from build123d import *
from build123d.topology import SkipClean

# Parameters (mm, degrees)
SKETCH_1_R               = 12.75
EXTRUDE_1_DEPTH          = 7
EXTRUDE_START            = -2.3
SKETCH_1_3_R             = 12.75
SKETCH_1_3_R_2           = 9.75
EXTRUDE_2_DEPTH          = 2.3
EXTRUDE_3_DEPTH          = 3.3
FILLET_1_R               = 1
EXTRUDE_4_DEPTH          = 3.3
CUT_EXTRUDE_1_REACH      = 22.288
SKETCH_6_R               = 1.3500000000000005
SKETCH_6_R_2             = 1.5499999999999994
CUT_EXTRUDE_START        = -1
CUT_EXTRUDE_2_DEPTH      = 1
EXTRUDE_START_2          = 4.5
EXTRUDE_5_DEPTH          = 4.5
CUT_EXTRUDE_3_DEPTH      = 3
CUT_EXTRUDE_3_DEPTH_BACK = 25
SKETCH_17_R              = 2.5
SKETCH_17_R_2            = 2.5000000000000004
CUT_EXTRUDE_4_DEPTH      = 6.3
SKETCH_18_R              = 2.1
CUT_EXTRUDE_5_DEPTH      = 19.000000000000004


with BuildPart() as part:
    # 草图1 → 凸台-拉伸1 (new body)
    with BuildSketch(Plane(origin=(0, 0, 0), x_dir=(0, 0, -1), z_dir=(1, 0, 0))):
        Circle(SKETCH_1_R)
    extrude(amount=EXTRUDE_1_DEPTH)

    # 草图1<3> → 凸台-拉伸2 (add)
    with BuildSketch(Plane(origin=(0, 0, 0), x_dir=(0, 0, -1), z_dir=(1, 0, 0)).offset(EXTRUDE_START)):
        Circle(SKETCH_1_3_R)
        Circle(SKETCH_1_3_R_2, mode=Mode.SUBTRACT)
    extrude(amount=EXTRUDE_2_DEPTH)

    # 草图4 → 凸台-拉伸3 (add)
    with BuildSketch(Plane(origin=(7, 0, 0), x_dir=(0, 0, -1), z_dir=(1, 0, 0))):
        with BuildLine():
            Line((7.293731545630563, -1.9503794862215074), (5.5903528728314456, -1.4948876985254207))
            ThreePointArc((5.590352872831452, -1.4948876985253963), (4.450095710648993, -0.01722480337626947), (5.557231396787749, 1.4854144081735148))
            ThreePointArc((5.557231396787749, 1.4854144081735148), (5.599745988830406, 1.4974300406171406), (5.642585759719926, 1.508229114174971))
            Line((5.642585759719926, 1.5082291141749726), (7.293933423650666, 1.949624376989515))
            ThreePointArc((7.293933423650662, 1.949624376989514), (4.6e-16, 7.550000000000002), (-7.293933423650662, 1.949624376989515))
            Line((-7.293933423650666, 1.949624376989515), (-5.642585759719924, 1.5082291141749722))
            ThreePointArc((-5.642585759719924, 1.5082291141749706), (-5.599745988830406, 1.4974300406171406), (-5.557231396787749, 1.4854144081735148))
            ThreePointArc((-5.557231396787749, 1.4854144081735148), (-4.757262832498563, 0.9263392102844973), (-4.449999999999999, 0))
            ThreePointArc((-4.449999999999999, -3.8e-16), (-4.767633770522892, -0.9400922701758461), (-5.590352872831452, -1.4948876985253963))
            Line((-5.5903528728314456, -1.4948876985254207), (-7.293731545630563, -1.9503794862215074))
            ThreePointArc((-7.2937315456305605, -1.950379486221506), (-1.39e-15, -7.550000000000002), (7.2937315456305605, -1.9503794862215056))
        make_face()
        with BuildLine():
            ThreePointArc((-0.9205316546017519, -3.4285742624123157), (-1.7750000000000141, -3.074390183434749), (-2.5089665827097076, -2.5114909290789753))
            ThreePointArc((-2.5089665827097076, -2.5114909290789753), (-2.5295691102475106, -2.490738869589025), (-2.55, -2.4698178070456938))
            Line((-2.55, -2.4698178070456938), (-2.55, 0))
            Line((-2.55, 0), (-2.55, 2.4698178070456938))
            ThreePointArc((-2.55, 2.469817807045694), (2.2e-16, 3.5499999999999994), (2.55, 2.4698178070456938))
            Line((2.55, 2.4698178070456938), (2.55, -1.2e-16))
            Line((2.55, -1.2e-16), (2.55, -2.4698178070456938))
            ThreePointArc((2.549999999999999, -2.4698178070456946), (0.9453016753082151, -3.4218276903811913), (-0.9205316546017519, -3.4285742624123157))
        make_face(mode=Mode.SUBTRACT)
    extrude(amount=EXTRUDE_3_DEPTH)

    # 圆角1
    fillet_1_edges = [part.edges().sort_by_distance(p)[0] for p in [
        (7, 1.56e-15, 12.75),
    ]]
    fillet(fillet_1_edges, radius=FILLET_1_R)

    # 草图5 → 凸台-拉伸4 (add)
    with BuildSketch(Plane(origin=(7, 0, 0), x_dir=(0, 0, -1), z_dir=(1, 0, 0))):
        with BuildLine():
            ThreePointArc((5.65345654698472, -1.3047634403110198), (4.6499999999999995, 1.7e-16), (5.65345654698472, 1.3047634403110198))
            Line((5.65345654698472, 1.3047634403110195), (7.3500000000000005, 1.7553631492193538))
            Line((7.3500000000000005, 1.7553631492193538), (7.293933423650666, 1.9496243769895145))
            Line((7.293933423650666, 1.9496243769895145), (5.642585759719882, 1.5082291141749606))
            ThreePointArc((5.642585759719882, 1.5082291141749606), (4.4500975021885605, 0.01738526036219645), (5.60884432582712, -1.499832403491257))
            Line((5.60884432582712, -1.499832403491257), (7.293731545630563, -1.950379486221502))
            Line((7.293731545630563, -1.950379486221502), (7.3500000000000005, -1.7595376594411802))
            Line((7.3500000000000005, -1.7595376594411802), (5.65345654698472, -1.3047634403110195))
        make_face()
    extrude(amount=EXTRUDE_4_DEPTH)

    # 草图6 → 切除-拉伸1 (cut, up to next)
    with BuildSketch(Plane(origin=(7, 0, 0), x_dir=(0, 0, -1), z_dir=(1, 0, 0)), mode=Mode.PRIVATE) as cut_extrude_1_sk1:
        with Locations(Location((6, 0, 0), (0, 0, 255.125726416))):
            Circle(SKETCH_6_R)
    cut_extrude_1_tool1 = extrude(cut_extrude_1_sk1.sketch, amount=-CUT_EXTRUDE_1_REACH, mode=Mode.PRIVATE) & part.part
    # 草图6 → 切除-拉伸1 (cut, up to next)
    with BuildSketch(Plane(origin=(7, 0, 0), x_dir=(0, 0, -1), z_dir=(1, 0, 0)), mode=Mode.PRIVATE) as cut_extrude_1_sk2:
        with Locations(Location((-6, -7.3e-16, 0), (0, 0, 76.668199875))):
            Circle(SKETCH_6_R_2)
    cut_extrude_1_tool2 = extrude(cut_extrude_1_sk2.sketch, amount=-CUT_EXTRUDE_1_REACH, mode=Mode.PRIVATE) & part.part
    add(cut_extrude_1_tool1.solids().sort_by_distance((7, 0, -6))[0], mode=Mode.SUBTRACT)
    add(cut_extrude_1_tool2.solids().sort_by_distance((7, 0, 6))[0], mode=Mode.SUBTRACT)

    # 草图7 → 切除-拉伸2 (cut)
    with BuildSketch(Plane(origin=(7, 0, 0), x_dir=(0, 0, -1), z_dir=(1, 0, 0)).offset(CUT_EXTRUDE_START)):
        with BuildLine():
            Line((2.55, -2.4698178070456938), (2.55, 2.4698178070456938))
            ThreePointArc((2.55, 2.4698178070456938), (2.2e-16, 3.55), (-2.55, 2.4698178070456938))
            Line((-2.55, 2.4698178070456938), (-2.55, -2.4698178070456938))
            ThreePointArc((-2.55, -2.4698178070456938), (2.2e-16, -3.55), (2.55, -2.4698178070456938))
        make_face()
    extrude(amount=CUT_EXTRUDE_2_DEPTH, mode=Mode.SUBTRACT)

    # 草图9 → 凸台-拉伸5 (add)
    with SkipClean():  # the faces are left unmerged after this step: merging them gives an invalid solid
        with BuildSketch(Plane.ZY.offset(2.3).offset(EXTRUDE_START_2)):
            with BuildLine():
                ThreePointArc((-3.4999999999999996, 10.25), (-3.3535533905932735, 9.896446609406727), (-3, 9.75))
                Line((-3, 9.75), (3, 9.75))
                ThreePointArc((3, 9.75), (3.3535533905932735, 9.896446609406727), (3.5000000000000004, 10.25))
                Line((3.5, 10.25), (3.5, 12.260199835239227))
                ThreePointArc((3.5000000000000004, 12.260199835239227), (1e-15, 12.75), (-3.5, 12.260199835239227))
                Line((-3.5, 12.260199835239227), (-3.5, 10.25))
            make_face()
            with BuildLine():
                Line((-3.5, -10.25), (-3.5, -12.260199835239227))
                ThreePointArc((-3.5, -12.260199835239227), (1e-15, -12.75), (3.5000000000000004, -12.260199835239227))
                Line((3.5, -12.260199835239227), (3.5, -10.25))
                ThreePointArc((3.5000000000000004, -10.25), (3.3535533905932735, -9.896446609406727), (3, -9.75))
                Line((3, -9.75), (-3, -9.75))
                ThreePointArc((-3, -9.75), (-3.3535533905932735, -9.896446609406727), (-3.4999999999999996, -10.25))
            make_face()
        extrude(amount=-EXTRUDE_5_DEPTH)

    # 草图16 → 切除-拉伸3 (cut, two sides: drawn at the far end of the back side and taken through both)
    with BuildSketch(Plane(origin=(0, 9.75, 0), x_dir=(1, 0, 0), z_dir=(0, 1, 0)).offset(-CUT_EXTRUDE_3_DEPTH_BACK)):
        with BuildLine():
            Line((-3.797155055625174, 1.499995743144704), (-3.8000000000000003, 1.499998441052766))
            ThreePointArc((-3.8000000000000003, 1.499998441052766), (-5.299998441052766, 3.3e-16), (-3.8000000000000007, -1.4999984410527665))
            Line((-3.8000000000000003, -1.4999984410527663), (-3.7988775259417356, -1.4999980210696007))
            Line((-3.7988775259417356, -1.4999980210696007), (-2.8462661595831507, -1.4996415934672602))
            ThreePointArc((-2.8462661595831507, -1.4996415934672602), (-1.300658265078132, -0.05513463794275678), (-2.735998812247351, 1.4989894310320704))
            Line((-2.735998812247351, 1.49898943103207), (-2.8611580419850906, 1.4991081216110296))
            Line((-2.8611580419850906, 1.4991081216110296), (-3.797155055625174, 1.499995743144704))
        make_face()
    extrude(amount=CUT_EXTRUDE_3_DEPTH + CUT_EXTRUDE_3_DEPTH_BACK, mode=Mode.SUBTRACT)

    # 草图17 → 切除-拉伸4 (cut)
    with SkipClean():  # the faces are left unmerged after this step: merging them gives an invalid solid
        with BuildSketch(Plane(origin=(10.3, 0, 0), x_dir=(0, 0, -1), z_dir=(1, 0, 0))):
            with Locations((-6, 0)):
                Circle(SKETCH_17_R)
            with Locations((6, 0)):
                Circle(SKETCH_17_R_2)
        extrude(amount=-CUT_EXTRUDE_4_DEPTH, mode=Mode.SUBTRACT)

    # 草图18 → 切除-拉伸5 (cut)
    with SkipClean():  # the faces are left unmerged after this step: merging them gives an invalid solid
        with BuildSketch(Plane(origin=(10.3, 0, 0), x_dir=(0, 0, -1), z_dir=(1, 0, 0))):
            Circle(SKETCH_18_R)
        extrude(amount=-CUT_EXTRUDE_5_DEPTH, mode=Mode.SUBTRACT)


solid = part.part
Could you check a few things on this model? Use its own coordinates, in mm. A direction names the side the tool comes from. Round coordinates to 2 decimals unless told otherwise and drop trailing zeros. Order: outer loops, then holes, each group sorted by start corner. A loop starts at its lowest first (then second) coordinate and runs counter-clockwise, first axis right, second up.
Q1. Imagine slicing it at A-A, the plane y = 0. State how many separate pieces and enclosed holes the cut face has, then the cut area to 3 significant figures.
Geometry says:
separate pieces: 4
enclosed holes: 0
area: 115 mm2
Q2. Please list where these lines run through material, in increasing order: probe 1 along Z at (x, y) = (7.5, 0); probe 2 along X at (y, z) = (5.25, 5.5); probe 3 along X at (y, z) = (1, 10.5).
Geometry says:
probe 1: z = -3.5 to -2.55, 2.55 to 3.5
probe 2: x = 0 to 7
probe 3: x = -2.3 to 7
Q3. Imagine slicing it at D-D, the plane x = 3.5. List the corners of the cut face in (y, z) for me.
Geometry says:
outline: circle Ø25.5 at (0, 0); hole circle Ø4.2 at (0, 0); hole circle Ø3.1 at (0, 6); hole circle Ø2.7 at (0, -6)
Q4. Thinking about a two-plate mould opening in X: for faces 1 (the face through (7.2, -1.5, -4)), 2 (the face through (-2.3, -1, -10)), 3 (the face through (6, -2, -2)), 4 (the face through (-5.3, 11.2, 0)), which applies, released by +X, released by -X, zero draft, split by the parting line, or undercut?
Geometry says:
face 1: zero draft
face 2: released by -X
face 3: released by +X
face 4: undercut
Q5. I'm going to push flat-ended pins straight in: P1, Ø3, axis at y = 6, z = 5.5, coming from the -X side; P2, Ø3, axis at x = 2.5, y = -9, coming from the +Z side; P3, Ø4, axis at y = 0, z = 6, coming from the +X side. Where does each tip first touch, or does it pass through?
Geometry says:
P1: stops at x = 0
P2: stops at z = 10.31
P3: stops at x = 4
Q6. Which directions (+Z, -Z, +X, -X, +Y, -Y) give clear straight access to the entire face, cutting with the end or side of a thin tool? Please do faces 5 (the face through (8, 0, 2.55)), 6 (the face through (-1.17, -8.65, -4.5)), 7 (the face through (8.63, 7.55, -0.14)), 8 (the face through (-1.302, 11.177, 0.088)), 9 (the face through (-5, -11, -3.5)).
Geometry says:
face 5: +X
face 6: -X
face 7: +X, +Y
face 8: +Y, -Y
face 9: -Z, -X, +Y, -Y
Q7. Imagine slicing it at C-C, the plane x = -4.75. List the corners of the cut face in (y, z) for me, then the cut area to 3 significant figures.
Geometry says:
outline: (-12.7, -1.16) arc R12.75 ccw to (-12.26, -3.5) - (-10.25, -3.5) arc R0.5 ccw to (-9.75, -3) - (-9.75, -1.16) - close; (-12.7, 1.16) - (-9.75, 1.16) - (-9.75, 3) arc R0.5 ccw to (-10.25, 3.5) - (-12.26, 3.5) arc R12.75 ccw to start; (9.75, -3) arc R0.5 ccw to (10.25, -3.5) - (12.26, -3.5) arc R12.75 ccw to (12.7, -1.16) - (9.75, -1.16) - close; (9.75, 1.16) - (12.7, 1.16) arc R12.75 ccw to (12.26, 3.5) - (10.25, 3.5) arc R0.5 ccw to (9.75, 3) - close
area: 25.7 mm2
